from build123d import *

# Parameters (mm, degrees)
SKETCH_1_W          = 94
SKETCH_1_H          = 48
EXTRUDE_1_DEPTH     = 1
SKETCH_2_W          = 8
SKETCH_2_H          = 10
EXTRUDE_2_DEPTH     = 2
FILLET_1_R          = 10
SKETCH_3_R          = 1.5
CUT_EXTRUDE_1_DEPTH = 71.802542327
FILLET_2_R          = 2


with BuildPart() as part:
    # Эскиз1 → Бобышка-Вытянуть1 (new body)
    with BuildSketch(Plane.XY):
        Rectangle(SKETCH_1_W, SKETCH_1_H)
    extrude(amount=EXTRUDE_1_DEPTH)

    # Эскиз2 → Бобышка-Вытянуть2 (add)
    with BuildSketch(Plane.XZ.offset(24)):
        with Locations((-28, 5)):
            Rectangle(SKETCH_2_W, SKETCH_2_H)
        with Locations((28, 5)):
            Rectangle(SKETCH_2_W, SKETCH_2_H)
        with Locations((0, 5)):
            Rectangle(SKETCH_2_W, SKETCH_2_H)
    extrude_2 = extrude(amount=EXTRUDE_2_DEPTH)

    # Зеркальное отражение1: Бобышка-Вытянуть2 across plane
    add(extrude_2.mirror(Plane.ZX))

    # Скругление1
    # the kernel refuses this fillet: 10 mm, written as the material it adds along each edge
    with BuildSketch(Plane(origin=(-32, 24, 1), x_dir=(-1, 0, 0), z_dir=(0, 0, -1)), Plane(origin=(-24, 24, 0), x_dir=(1, 0, 0), z_dir=(0, 0, 1)), Plane(origin=(-4, 24, 1), x_dir=(-1, 0, 0), z_dir=(0, 0, -1)), Plane(origin=(4, 24, 0), x_dir=(1, 0, 0), z_dir=(0, 0, 1)), Plane(origin=(24, 24, 1), x_dir=(-1, 0, 0), z_dir=(0, 0, -1)), Plane(origin=(32, 24, 0), x_dir=(1, 0, 0), z_dir=(0, 0, 1))) as fillet_1_piece_1:
        with BuildLine():
            CenterArc((6, 10), FILLET_1_R, 233.130102354, 36.869897646)
            Line((0, 2), (0, 0))
            Line((0, 0), (6, 0))
        make_face()
    extrude(amount=1)
    with BuildSketch(Plane(origin=(32, -24, 0), x_dir=(0, -1, 0), z_dir=(0, 0, 1)), Plane(origin=(4, -24, 0), x_dir=(0, -1, 0), z_dir=(0, 0, 1)), Plane(origin=(-24, -24, 0), x_dir=(0, -1, 0), z_dir=(0, 0, 1))) as fillet_1_piece_2:
        with BuildLine():
            CenterArc((10, 6), FILLET_1_R, 180, 36.869897646)
            Line((0, 6), (0, 0))
            Line((0, 0), (2, 0))
        make_face()
    extrude(amount=1)
    with BuildSketch(Plane(origin=(24, -24, 1), x_dir=(-1, 0, 0), z_dir=(0, 0, -1)), Plane(origin=(-4, -24, 1), x_dir=(-1, 0, 0), z_dir=(0, 0, -1)), Plane(origin=(-32, -24, 1), x_dir=(-1, 0, 0), z_dir=(0, 0, -1))) as fillet_1_piece_3:
        with BuildLine():
            CenterArc((6, -10), FILLET_1_R, 90, 36.869897646)
            Line((0, -2), (0, 0))
            Line((0, 0), (6, 0))
        make_face()
    extrude(amount=1)

    # Эскиз3 → Вырез-Вытянуть1 (cut, through all)
    with BuildSketch(Plane.XZ.offset(26)):
        with Locations(Location((-28, 6, 0), (0, 0, 270))):
            Circle(SKETCH_3_R)
        with Locations(Location((0, 6, 0), (0, 0, 270))):
            Circle(SKETCH_3_R)
        with Locations(Location((28, 6, 0), (0, 0, 270))):
            Circle(SKETCH_3_R)
    extrude(amount=-CUT_EXTRUDE_1_DEPTH, mode=Mode.SUBTRACT)

    # Скругление2
    fillet_2_edges = [part.edges().sort_by_distance(p)[0] for p in [
        (47, -24, 0.5),
        (-47, -24, 0.5),
        (-47, 24, 0.5),
        (47, 24, 0.5),
    ]]
    fillet(fillet_2_edges, radius=FILLET_2_R)


solid = part.part
Check sheet for the modelled part. Datum: model origin and axes. Units: mm. A direction names the side the tool comes from. Round coordinates to 2 decimals unless told otherwise and drop trailing zeros. Write each loop counter-clockwise with the first axis right and the second up, starting at its lowest first coordinate (ties: lowest second). Pieces come first, ordered by that corner, then holes. Notation, with made-up numbers: (42, -10) -> (54, -10) arc R17 ccw to (54, -6) -> close; hole circle Ø9 at (62.5, -26). An arc over 180 degrees is marked (long way). Answer as CSV lines item,"result". Start each with the question number.
1) Section check A-A on x = -28. Enter the section's corners in (y, z).
2) Release check for a two-part mould opening along X. For faces 4 (the flat face through (24, 25, 5)), 5 (the cylindrical face through (46.4, -23.43, 0.51)), 6 (the cylindrical face through (-26.513, 24.986, 6.195)), 7 (the flat face through (28, 26, 4)) record: pulls with the +X half, pulls with the -X half, needs draft (parallel to the pull), parting line crosses it, or undercut.
3) Section check D-D on y = -18.5. Enter the section's corners in (x, z).
4) Section check C-C on x = 30.5. Enter the section's corners in (y, z), and give its area (3 significant figures).
5) Tool access check on faces 1 (the flat face through (32, -25, 5)), 2 (the flat face through (-4, 25, 5)), 3 (the cylindrical face through (21.205, 24.528, 0.507)). Record the directions out of +Z, -Z, +X, -X, +Y, -Y that give a thin tool (end or side, any length) a straight path to the whole face; none if there is none.
6) Material ranges on line 1 (X direction, y = -25.15, z = 6); line 2 (Y direction, x = -26, z = 4.75); line 3 (Z direction, x = 22.5, y = -4), recorded low to high. Write a range as from..to.
7) Go/stop test with flat-tipped pins: P1, Ø1.6, axis at y = 25, z = 3.5, coming from the +X side; P2, Ø0.8, axis at x = -16, z = 0.5, coming from the -Y side; P3, Ø0.5, axis at x = -14, z = 0.5, coming from the +Y side. Record where each tip stops, or that it passes through.
8) Section check B-B on z = 3. Enter the section's corners in (x, y).
Found:
1,outline,"(-26, 0) -> (26, 0) -> (26, 4.5) -> (24, 4.5) -> (24, 1) -> (-24, 1) -> (-24, 4.5) -> (-26, 4.5) -> close; (-26, 7.5) -> (-24, 7.5) -> (-24, 10) -> (-26, 10) -> close; (24, 7.5) -> (26, 7.5) -> (26, 10) -> (24, 10) -> close"
2,face 4,"undercut"
2,face 5,"pulls with the +X half"
2,face 6,"undercut"
2,face 7,"needs draft"
3,outline,"(-47, 0) -> (47, 0) -> (47, 1) -> (-47, 1) -> close"
4,outline,"(-26, 0) -> (26, 0) -> (26, 10) -> (24, 10) -> (24, 1) -> (-24, 1) -> (-24, 10) -> (-26, 10) -> close"
4,area,"88.0 mm^2"
5,face 1,"+Z, +X, +Y, -Y"
5,face 2,"+Z, +Y, -Y"
5,face 3,"+Z, -Z, +Y"
6,line 1,"x = -32..-29.5, -26.5..-24, -4..-1.5, 1.5..4, 24..26.5, 29.5..32"
6,line 2,"y = -26..-24, 24..26"
6,line 3,"z = 0..1"
7,P1,"stops at x = 32"
7,P2,"stops at y = -24"
7,P3,"stops at y = 24"
8,outline,"(-32, -26) -> (-24, -26) -> (-24, -24) -> (-32, -24) -> close; (-32, 24) -> (-24, 24) -> (-24, 26) -> (-32, 26) -> close; (-4, -26) -> (4, -26) -> (4, -24) -> (-4, -24) -> close; (-4, 24) -> (4, 24) -> (4, 26) -> (-4, 26) -> close; (24, -26) -> (32, -26) -> (32, -24) -> (24, -24) -> close; (24, 24) -> (32, 24) -> (32, 26) -> (24, 26) -> close"
